Input: part model. Units: mm. Frame: model coordinates. A direction names the side the tool comes from. Give positions to 0.01 mm unless a question says otherwise; leave off trailing zeros. Write each loop counter-clockwise with the first axis right and the second up, starting at its lowest first coordinate (ties: lowest second). Pieces come first, ordered by that corner, then holes.
```python
from build123d import *

# Parameters (mm, degrees)
SKETCH1_W            = 65
SKETCH1_H            = 33
BOSS_EXTRUDE1_DEPTH  = 2
SKETCH2_W            = 65
SKETCH2_H            = 33
SKETCH2_W_2          = 61
SKETCH2_H_2          = 29
BOSS_EXTRUDE2_DEPTH  = 21
SKETCH3_W            = 50.5
SKETCH3_H            = 29
BOSS_EXTRUDE3_DEPTH  = 11
SKETCH4_R            = 3
CUT_EXTRUDE1_DEPTH   = 2
SKETCH5_W            = 4
SKETCH5_H            = 6
BOSS_EXTRUDE4_DEPTH  = 9.5
SKETCH6_W            = 4
SKETCH6_H            = 6
BOSS_EXTRUDE5_DEPTH  = 9.5
SKETCH7_W            = 3
SKETCH7_H            = 4
BOSS_EXTRUDE8_DEPTH  = 9.5
SKETCH9_W            = 3
SKETCH9_H            = 4
BOSS_EXTRUDE9_DEPTH  = 9.5
SKETCH10_W           = 3
SKETCH10_H           = 4
BOSS_EXTRUDE10_DEPTH = 9.5
SKETCH11_W           = 2
SKETCH11_H           = 29
CUT_EXTRUDE2_DEPTH   = 3
SKETCH13_W           = 31
SKETCH13_H           = 2
CUT_EXTRUDE3_DEPTH   = 63
SKETCH14_W           = 15
SKETCH14_H           = 1.5
BOSS_EXTRUDE11_DEPTH = 5
SKETCH15_W           = 15
SKETCH15_H           = 1.5
BOSS_EXTRUDE12_DEPTH = 5
SKETCH16_W           = 14.920438195
SKETCH16_H           = 1
BOSS_EXTRUDE13_DEPTH = 5
SKETCH17_W           = 15
SKETCH17_H           = 1
BOSS_EXTRUDE14_DEPTH = 5
SKETCH18_W           = 15
SKETCH18_H           = 4
BOSS_EXTRUDE15_DEPTH = 5
SKETCH19_W           = 18
SKETCH19_H           = 29
BOSS_EXTRUDE16_DEPTH = 7
SKETCH20_W           = 20
SKETCH20_H           = 2.5
CUT_EXTRUDE4_DEPTH   = 6
SKETCH21_W           = 20
SKETCH21_H           = 2.5
CUT_EXTRUDE5_DEPTH   = 6
SKETCH22_W           = 20
SKETCH22_H           = 2.5
CUT_EXTRUDE6_DEPTH   = 6
SKETCH23_W           = 20
SKETCH23_H           = 2.5
CUT_EXTRUDE7_DEPTH   = 6


with BuildPart() as part:
    # Sketch1 → Boss-Extrude1 (new body)
    with BuildSketch(Plane(origin=(0, 0, 0), x_dir=(1, 0, 0), z_dir=(0, 1, 0))):
        Rectangle(SKETCH1_W, SKETCH1_H)
    extrude(amount=BOSS_EXTRUDE1_DEPTH)

    # Sketch2 → Boss-Extrude2 (add)
    with BuildSketch(Plane(origin=(0, 2, 0), x_dir=(1, 0, 0), z_dir=(0, 1, 0))):
        Rectangle(SKETCH2_W, SKETCH2_H)
        Rectangle(SKETCH2_W_2, SKETCH2_H_2, mode=Mode.SUBTRACT)
    extrude(amount=BOSS_EXTRUDE2_DEPTH)

    # Sketch3 → Boss-Extrude3 (add)
    with BuildSketch(Plane(origin=(0, 2, 0), x_dir=(1, 0, 0), z_dir=(0, 1, 0))):
        with Locations((-5.25, 0)):
            Rectangle(SKETCH3_W, SKETCH3_H)
    extrude(amount=BOSS_EXTRUDE3_DEPTH)

    # Sketch4 → Cut-Extrude1 (cut)
    with BuildSketch(Plane(origin=(0, 2, 0), x_dir=(1, 0, 0), z_dir=(0, 1, 0))):
        with Locations((26.5, 0)):
            Circle(SKETCH4_R)
    extrude(amount=-CUT_EXTRUDE1_DEPTH, mode=Mode.SUBTRACT)

    # Sketch5 → Boss-Extrude4 (add)
    with BuildSketch(Plane(origin=(0, 2, 0), x_dir=(1, 0, 0), z_dir=(0, 1, 0))):
        with Locations((22, 11.5)):
            Rectangle(SKETCH5_W, SKETCH5_H)
    extrude(amount=BOSS_EXTRUDE4_DEPTH)

    # Sketch6 → Boss-Extrude5 (add)
    with BuildSketch(Plane(origin=(0, 2, 0), x_dir=(1, 0, 0), z_dir=(0, 1, 0))):
        with Locations((22, -11.5)):
            Rectangle(SKETCH6_W, SKETCH6_H)
    extrude(amount=BOSS_EXTRUDE5_DEPTH)

    # Sketch7 → Boss-Extrude8 (add)
    with BuildSketch(Plane(origin=(0, 2, 0), x_dir=(1, 0, 0), z_dir=(0, 1, 0))):
        with Locations((29, 6)):
            Rectangle(SKETCH7_W, SKETCH7_H)
    extrude(amount=BOSS_EXTRUDE8_DEPTH)

    # Sketch9 → Boss-Extrude9 (add)
    with BuildSketch(Plane(origin=(0, 2, 0), x_dir=(1, 0, 0), z_dir=(0, 1, 0))):
        with Locations((29, -6)):
            Rectangle(SKETCH9_W, SKETCH9_H)
    extrude(amount=BOSS_EXTRUDE9_DEPTH)

    # Sketch10 → Boss-Extrude10 (add)
    with BuildSketch(Plane(origin=(0, 2, 0), x_dir=(1, 0, 0), z_dir=(0, 1, 0))):
        with Locations((21.5, 0)):
            Rectangle(SKETCH10_W, SKETCH10_H)
    extrude(amount=BOSS_EXTRUDE10_DEPTH)

    # Sketch11 → Cut-Extrude2 (cut)
    with BuildSketch(Plane(origin=(0, 23, 0), x_dir=(1, 0, 0), z_dir=(0, 1, 0))):
        with Locations((-31.5, 0)):
            Rectangle(SKETCH11_W, SKETCH11_H)
    extrude(amount=-CUT_EXTRUDE2_DEPTH, mode=Mode.SUBTRACT)

    # Sketch13 → Cut-Extrude3 (cut)
    with BuildSketch(Plane.ZY.offset(32.5)):
        with Locations((0, 21)):
            Rectangle(SKETCH13_W, SKETCH13_H)
    extrude(amount=-CUT_EXTRUDE3_DEPTH, mode=Mode.SUBTRACT)

    # Sketch14 → Boss-Extrude11 (add)
    with BuildSketch(Plane(origin=(0, 13, 0), x_dir=(1, 0, 0), z_dir=(0, 1, 0))):
        with Locations((7.5, 13.75)):
            Rectangle(SKETCH14_W, SKETCH14_H)
    extrude(amount=BOSS_EXTRUDE11_DEPTH)

    # Sketch15 → Boss-Extrude12 (add)
    with BuildSketch(Plane(origin=(0, 13, 0), x_dir=(1, 0, 0), z_dir=(0, 1, 0))):
        with Locations((7.5, -13.75)):
            Rectangle(SKETCH15_W, SKETCH15_H)
    extrude(amount=BOSS_EXTRUDE12_DEPTH)

    # Sketch16 → Boss-Extrude13 (add)
    with BuildSketch(Plane(origin=(0, 13, 0), x_dir=(1, 0, 0), z_dir=(0, 1, 0))):
        with Locations((7.539780903, 7.5)):
            Rectangle(SKETCH16_W, SKETCH16_H)
    extrude(amount=BOSS_EXTRUDE13_DEPTH)

    # Sketch17 → Boss-Extrude14 (add)
    with BuildSketch(Plane(origin=(0, 13, 0), x_dir=(1, 0, 0), z_dir=(0, 1, 0))):
        with Locations((7.5, -7.5)):
            Rectangle(SKETCH17_W, SKETCH17_H)
    extrude(amount=BOSS_EXTRUDE14_DEPTH)

    # Sketch18 → Boss-Extrude15 (add)
    with BuildSketch(Plane(origin=(0, 13, 0), x_dir=(1, 0, 0), z_dir=(0, 1, 0))):
        with Locations((7.5, 0)):
            Rectangle(SKETCH18_W, SKETCH18_H)
    extrude(amount=BOSS_EXTRUDE15_DEPTH)

    # Sketch19 → Boss-Extrude16 (add)
    with BuildSketch(Plane(origin=(0, 13, 0), x_dir=(1, 0, 0), z_dir=(0, 1, 0))):
        with Locations((-21.5, 0)):
            Rectangle(SKETCH19_W, SKETCH19_H)
    extrude(amount=BOSS_EXTRUDE16_DEPTH)

    # Sketch20 → Cut-Extrude4 (cut)
    with BuildSketch(Plane(origin=(0, 20, 0), x_dir=(1, 0, 0), z_dir=(0, 1, 0))):
        with Locations((-22.5, 10.5)):
            Rectangle(SKETCH20_W, SKETCH20_H)
    extrude(amount=-CUT_EXTRUDE4_DEPTH, mode=Mode.SUBTRACT)

    # Sketch21 → Cut-Extrude5 (cut)
    with BuildSketch(Plane(origin=(0, 20, 0), x_dir=(1, 0, 0), z_dir=(0, 1, 0))):
        with Locations((-22.5, -10.5)):
            Rectangle(SKETCH21_W, SKETCH21_H)
    extrude(amount=-CUT_EXTRUDE5_DEPTH, mode=Mode.SUBTRACT)

    # Sketch22 → Cut-Extrude6 (cut)
    with BuildSketch(Plane(origin=(0, 20, 0), x_dir=(1, 0, 0), z_dir=(0, 1, 0))):
        with Locations((-22.5, 4.5)):
            Rectangle(SKETCH22_W, SKETCH22_H)
    extrude(amount=-CUT_EXTRUDE6_DEPTH, mode=Mode.SUBTRACT)

    # Sketch23 → Cut-Extrude7 (cut)
    with BuildSketch(Plane(origin=(0, 20, 0), x_dir=(1, 0, 0), z_dir=(0, 1, 0))):
        with Locations((-22.5, -4.5)):
            Rectangle(SKETCH23_W, SKETCH23_H)
    extrude(amount=-CUT_EXTRUDE7_DEPTH, mode=Mode.SUBTRACT)


solid = part.part
```
Q1. Pin query (flat end, axial travel): pin 1 (1 mm diameter, centred on x = -19.5, z = 8, fed in from +Y); pin 2 (12 mm diameter, centred on x = -19, z = -5.5, fed in from -Y); pin 3 (1.2 mm diameter, centred on x = -23.5, z = 10, fed in from +Y); pin 4 (3 mm diameter, centred on x = 19.5, z = -1.5, fed in from +Y). Return the tip coordinate at first contact, or that it passes through.
Q2. Material intervals for line 1 along Z through (x, y) = (28.5, 4); line 2 along Z through (x, y) = (-23.5, 19); line 3 along Z through (x, y) = (3.5, 17.5), sorted ascending.
Q3. Section C-C, the plane z = -11. Return the cut outline in (x, y).
Q4. Access query for faces 1 (the cylindrical face through (23.5, 1, -0.1)), 2 (the flat face through (-23, 17, -9.25)), 3 (the flat face through (24, 7, 12)). Directions: +Z, -Z, +X, -X, +Y, -Y. A direction counts if a zero-diameter tool reaches every point of the face in a straight line with its end or side. Return the directions, or none.
Q5. Section A-A, the plane x = 26.5. Return the cut outline in (y, z), then the cut area to 3 significant figures.
Q6. Section B-B, the plane z = 0. Return the cut outline in (x, y), then the cut area to 3 significant figures.
Q7. Mould query, pull axis Z, two halves, no side actions, for faces 4 (the flat face through (5, 23, 15)), 5 (the flat face through (0, 15, 14)). Classes: +Z half, -Z half, draft (parallel to the pull), parting line (faces both ways), or undercut.
Solutions:
1. pin 1: stops at y = 20
1. pin 2: stops at y = 0
1. pin 3: stops at y = 14
1. pin 4: stops at y = 13
2. line 1: z = -16.5 to -14.5, -8 to -4, 4 to 8, 14.5 to 16.5
2. line 2: z = -16.5 to -11.75, -9.25 to -5.75, -3.25 to 3.25, 5.75 to 9.25, 11.75 to 16.5
2. line 3: z = -16.5 to -13, -8 to -7, -2 to 2, 7 to 8, 13 to 16.5
3. outline: (-32.5, 0) - (32.5, 0) - (32.5, 23) - (30.5, 23) - (30.5, 2) - (24, 2) - (24, 11.5) - (20, 11.5) - (20, 13) - (-12.5, 13) - (-12.5, 14) - (-32.5, 14) - close
4. face 1: +Y, -Y
4. face 2: -X, +Y
4. face 3: +Y
5. outline: (0, -16.5) - (23, -16.5) - (23, -14.5) - (22, -14.5) - (22, -15.5) - (20, -15.5) - (20, -14.5) - (2, -14.5) - (2, -3) - (0, -3) - close; (0, 3) - (2, 3) - (2, 14.5) - (20, 14.5) - (20, 15.5) - (22, 15.5) - (22, 14.5) - (23, 14.5) - (23, 16.5) - (0, 16.5) - close
5. area: 134 mm2
6. outline: (-32.5, 0) - (23.5, 0) - (23.5, 2) - (23, 2) - (23, 11.5) - (20, 11.5) - (20, 13) - (15, 13) - (15, 18) - (0, 18) - (0, 13) - (-12.5, 13) - (-12.5, 20) - (-32.5, 20) - close; (29.5, 0) - (32.5, 0) - (32.5, 23) - (30.5, 23) - (30.5, 2) - (29.5, 2) - close
6. area: 981 mm2
7. face 4: draft
7. face 5: undercut
